Check sheet for the drawn part. Datum: minimum x, y, z corner. Units: mm. A direction names the side the tool comes from. Give positions to 0.01 mm unless a question says otherwise; leave off trailing zeros. Write each loop counter-clockwise with the first axis right and the second up, starting at its lowest first coordinate (ties: lowest second). Pieces come first, ordered by that corner, then holes. Notation, with made-up numbers: (-10.75, -7.75) - (34.25, -7.75) arc R17 ccw to (34.25, 2.25) - close; hole circle Ø6 at (-29, 46). An arc over 180 degrees is marked (long way). Answer as a JSON object with one key per item and string values. Group by question number.
Item 1: Sectioned sample at A-A, the plane z = 24.5. Record the boundary of the cut face in (x, y), and give its area (3 significant figures).
Item 2: Tool access check on the marked faces 4, 5, 6 and 7. Record the directions out of +Z, -Z, +X, -X, +Y, -Y that give a thin tool (end or side, any length) a straight path to the whole face; none if there is none.
Item 3: Sectioned sample at B-B, the plane y = 7.5. Record the boundary of the cut face in (x, z) (1 decimal), and give its area (3 significant figures).
Item 4: Sectioned sample at D-D, the plane y = 66.5. Record the boundary of the cut face in (x, z) (1 decimal).
Item 5: Draft check along Y on the marked faces 1, 2 and 3. Enter one of: +Y half, -Y half, draft (parallel to the pull), parting line (faces both ways), or undercut.
Item 6: Sectioned sample at C-C, the plane z = 4. Record the boundary of the cut face in (x, y).
Item 7: Scan lines: line 1 along X through (y, z) = (6, 5.5); line 2 along X through (y, z) = (16, 30); line 3 along Y through (x, z) = (89.5, 38). Record each from-to range of solid material in increasing order. Write a range as [from, to].
Item 8: Go/stop test with flat-tipped pins: pin 1 (8.5 mm diameter, centred on y = 6.57, z = 42.55, fed in from -X); pin 2 (6 mm diameter, centred on x = 51.5, z = 8.5, fed in from -Y); pin 3 (3.5 mm diameter, centred on x = 60, y = 70.5, fed in from +Z); pin 4 (16 mm diameter, centred on x = 42.5, y = 46.5, fed in from +Z) (1 decimal). Record where each tip stops, or that it passes through.
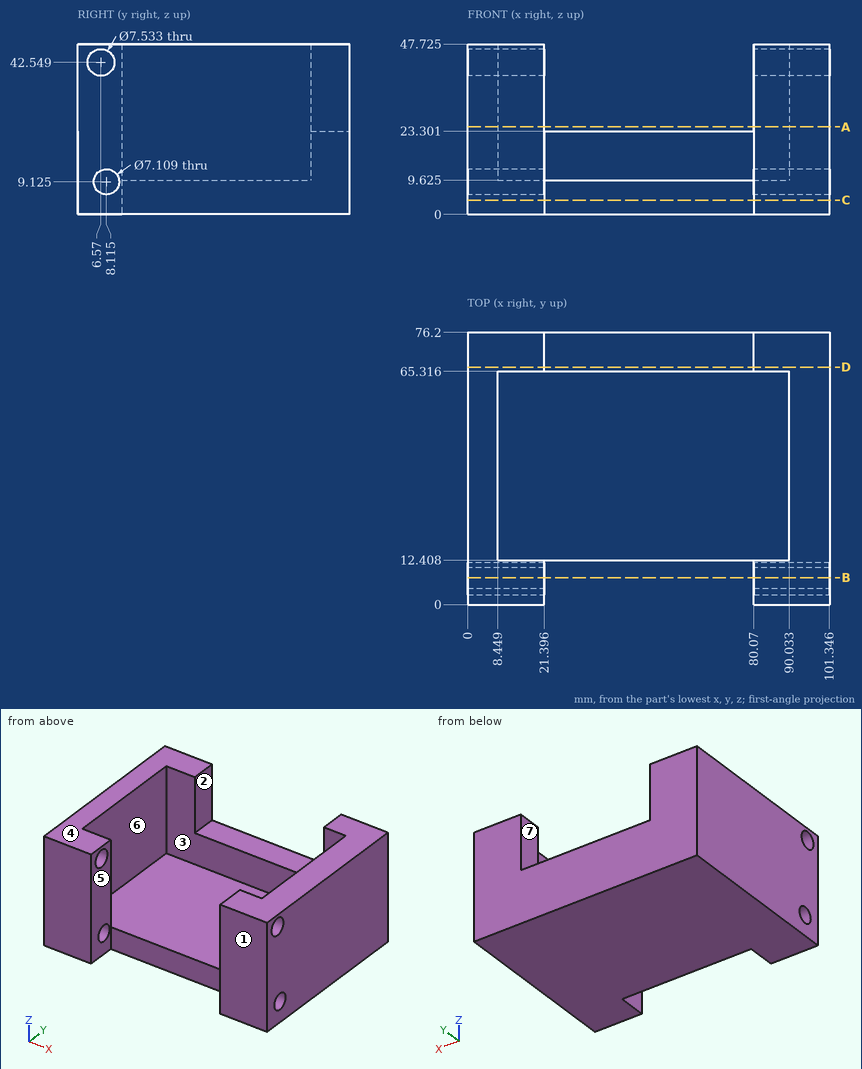
Geometry check:
{
 "1": {"outline": "(0, 0) - (21.4, 0) - (21.4, 12.41) - (8.45, 12.41) - (8.45, 65.32) - (21.4, 65.32) - (21.4, 76.2) - (0, 76.2) - close; (80.07, 0) - (101.35, 0) - (101.35, 76.2) - (80.07, 76.2) - (80.07, 65.32) - (90.03, 65.32) - (90.03, 12.41) - (80.07, 12.41) - close", "area": "2,040 mm^2"},
 "2": {"face 4": "+Z, +X, -X, +Y, -Y", "face 5": "+Z, -Z, -Y", "face 6": "+Z", "face 7": "+Z, +Y, -Y"},
 "3": {"outline": "(0, 0) - (21.4, 0) - (21.4, 5.6) - (0, 5.6) - close; (0, 12.6) - (21.4, 12.6) - (21.4, 38.9) - (0, 38.9) - close; (0, 46.2) - (21.4, 46.2) - (21.4, 47.7) - (0, 47.7) - close; (80.1, 0) - (101.3, 0) - (101.3, 5.6) - (80.1, 5.6) - close; (80.1, 12.6) - (101.3, 12.6) - (101.3, 38.9) - (80.1, 38.9) - close; (80.1, 46.2) - (101.3, 46.2) - (101.3, 47.7) - (80.1, 47.7) - close", "area": "1,430 mm^2"},
 "4": {"outline": "(0, 0) - (101.3, 0) - (101.3, 47.7) - (80.1, 47.7) - (80.1, 23.3) - (21.4, 23.3) - (21.4, 47.7) - (0, 47.7) - close"},
 "5": {"face 1": "-Y half", "face 2": "draft", "face 3": "undercut"},
 "6": {"outline": "(0, 0) - (21.4, 0) - (21.4, 12.41) - (80.07, 12.41) - (80.07, 0) - (101.35, 0) - (101.35, 76.2) - (0, 76.2) - close"},
 "7": {"line 1": "[0, 21.4], [80.07, 101.35]", "line 2": "[0, 8.45], [90.03, 101.35]", "line 3": "[0, 12.41], [65.32, 76.2]"},
 "8": {"pin 1": "x = 0", "pin 2": "y = 12.41", "pin 3": "z = 23.3", "pin 4": "z = 9.6"}
}
